from build123d import *

# Parameters (mm, degrees)
SKETCH_1_W          = 140
SKETCH_1_H          = 22
EXTRUDE_1_DEPTH     = 1
SKETCH_2_R          = 1.6
CUT_EXTRUDE_1_DEPTH = 10
CHAMFER_1_SIZE      = 10


with BuildPart() as part:
    # 草图1 → 凸台-拉伸1 (new body)
    with BuildSketch(Plane(origin=(0, 0, 0), x_dir=(1, 0, 0), z_dir=(0, 1, 0))):
        Rectangle(SKETCH_1_W, SKETCH_1_H)
    extrude(amount=EXTRUDE_1_DEPTH)

    # 草图2 → 切除-拉伸1 (cut)
    with BuildSketch(Plane.XZ):
        with Locations(Location((40, -6, 0), (0, 0, 270))):
            Circle(SKETCH_2_R)
        with Locations(Location((-40, -6, 0), (0, 0, 270))):
            Circle(SKETCH_2_R)
    extrude(amount=-CUT_EXTRUDE_1_DEPTH, mode=Mode.SUBTRACT)

    # 倒角1
    chamfer_1_edges = [part.edges().sort_by_distance(p)[0] for p in [
        (70, 0.5, 11),
        (-70, 0.5, 11),
    ]]
    chamfer(chamfer_1_edges, length=CHAMFER_1_SIZE)


solid = part.part
Verification items for the finished model (mm, model axes). Coordinates: 2 decimals unless noted, no trailing zeros. Write each loop counter-clockwise with the first axis right and the second up, starting at its lowest first coordinate (ties: lowest second). Pieces come first, ordered by that corner, then holes. Notation, with made-up numbers: M 27.5,48.25 L 60.5,48.25 A15 ccw 60.5,53.25 Z; hole C 71,47 d4. An arc over 180 degrees is marked long. Use CSV: the item, a comma, the result in double quotes.
Q1. Section check C-C, the plane y = 0.2. Enter the section's corners in (x, z).
Computed values:
outline,"M -70,-11 L 70,-11 L 70,1 L 60,11 L -60,11 L -70,1 Z; hole C -40,-6 d3.2; hole C 40,-6 d3.2"
Q2. Thickness scan on line 1 along X through (y, z) = (0.6, -6); line 2 along X through (y, z) = (0.4, -7); line 3 along X through (y, z) = (0.5, 6.5). Record the ranges inside material, lowest first. Write a range as [from, to].
Computed values:
line 1,"[-70, -41.6], [-38.4, 38.4], [41.6, 70]"
line 2,"[-70, -41.25], [-38.75, 38.75], [41.25, 70]"
line 3,"[-64.5, 64.5]"
Q3. Section check B-B, the plane x = -40. Enter the section's corners in (y, z).
Computed values:
outline,"M 0,-11 L 1,-11 L 1,-7.6 L 0,-7.6 Z; M 0,-4.4 L 1,-4.4 L 1,11 L 0,11 Z"
Q4. Mould release check, pull along X, two halves, no side actions. Record for faces 1 (the flat face through (-64.9, 0.5, 6.1)), 2 (the flat face through (-1, 1, 0)), 3 (the cylindrical face through (-41.42, 0.49, -6.74)): pulls with the +X half, pulls with the -X half, needs draft (parallel to the pull), parting line crosses it, or undercut.
Computed values:
face 1,"pulls with the -X half"
face 2,"needs draft"
face 3,"undercut"
Q5. Go/stop test with a flat-tipped pin: P1, Ø3.5, axis at x = -40, z = -6, coming from the -Y side. Record where the tip stops, or that it passes through.
Computed values:
P1,"y = 0"
Q6. Section check A-A, the plane z = -6. Enter the section's corners in (x, y), and give its area (3 significant figures).
Computed values:
outline,"M -70,0 L -41.6,0 L -41.6,1 L -70,1 Z; M -38.4,0 L 38.4,0 L 38.4,1 L -38.4,1 Z; M 41.6,0 L 70,0 L 70,1 L 41.6,1 Z"
area,"134 mm²"
